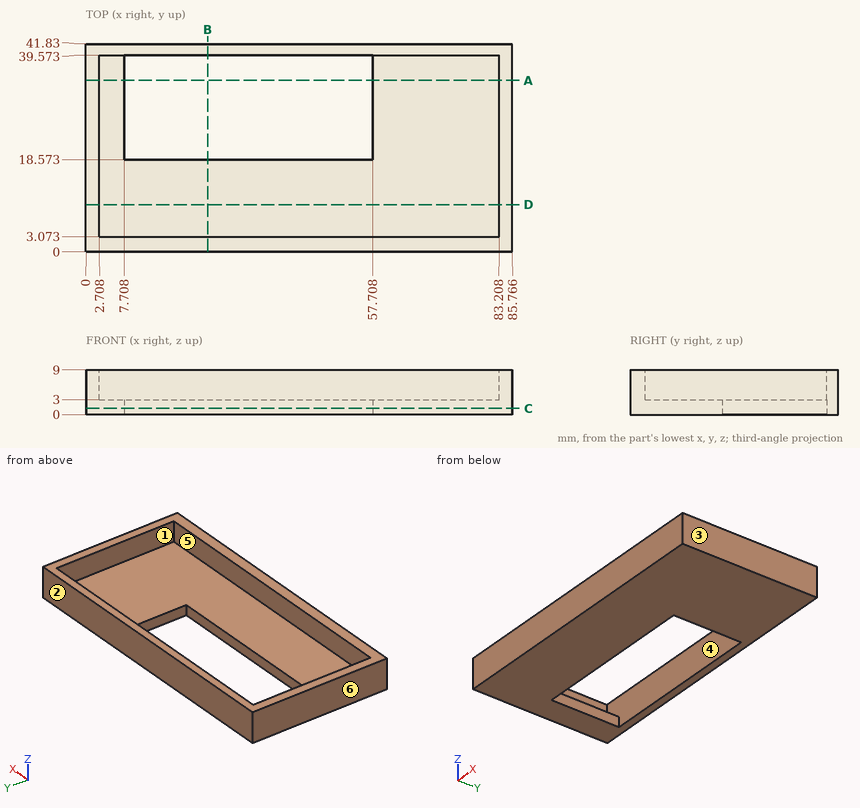
The figure shows three views and two pictorial views of one solid part (mm, origin at its lowest corner). Answer the questions. A direction names the side the tool comes from. Round coordinates to 2 decimals unless told otherwise and drop trailing zeros. Order: outer loops, then holes, each group sorted by start corner. A loop starts at its lowest first (then second) coordinate and runs counter-clockwise, first axis right, second up. Notation, with made-up numbers: (-40, -3.75) -> (6, -3.75) arc R16 cw to (6, 2.25) -> close; hole circle Ø9 at (7, 80.25). An arc over 180 degrees is marked (long way). Put each result on its own line as item: value.
Q1. Consider line 1 along X through (y, z) = (19, 7.5); line 2 along Y through (x, z) = (38.5, 7.5); line 3 along Y through (x, z) = (31.5, 1). Determine where each line is inside the solid, lowest interval first.
Results list:
line 1: 0 to 2.71, 83.21 to 85.77
line 2: 0 to 3.07, 39.57 to 41.83
line 3: 0 to 18.57, 39.57 to 41.83
Q2. Determine the mould class of the marked faces 3, 4, 5 and 6 for opening direction X: pulls with the +X half, pulls with the -X half, needs draft (parallel to the pull), parting line crosses it, or undercut.
Results list:
face 3: pulls with the +X half
face 4: undercut
face 5: undercut
face 6: pulls with the -X half
Q3. Section A-A, the plane y = 34.5 is taken. Write down the section's boundary in (x, z).
Results list:
outline: (0, 0) -> (7.71, 0) -> (7.71, 3) -> (2.71, 3) -> (2.71, 9) -> (0, 9) -> close; (57.71, 0) -> (85.77, 0) -> (85.77, 9) -> (83.21, 9) -> (83.21, 3) -> (57.71, 3) -> close
Q4. Section C-C, the plane z = 1.25 is taken. Write down the section's boundary in (x, y).
Results list:
outline: (0, 0) -> (85.77, 0) -> (85.77, 41.83) -> (0, 41.83) -> close; hole (7.71, 18.57) -> (57.71, 18.57) -> (57.71, 39.57) -> (7.71, 39.57) -> close
Q5. Section B-B, the plane x = 24.5 is taken. Write down the section's boundary in (y, z).
Results list:
outline: (0, 0) -> (18.57, 0) -> (18.57, 3) -> (3.07, 3) -> (3.07, 9) -> (0, 9) -> close; (39.57, 0) -> (41.83, 0) -> (41.83, 9) -> (39.57, 9) -> close
Q6. Which of the six approach directions +Z, -Z, +X, -X, +Y, -Y give full straight-line access (tool end or side, diameter ignored) to the marked faces 1 and 2?
Results list:
face 1: +Z
face 2: +Z, -Z, +X, -X, +Y
Q7. Section D-D, the plane y = 9.5 is taken. Write down the section's boundary in (x, z), and give its area (3 significant figures).
Results list:
outline: (0, 0) -> (85.77, 0) -> (85.77, 9) -> (83.21, 9) -> (83.21, 3) -> (2.71, 3) -> (2.71, 9) -> (0, 9) -> close
area: 289 mm^2
Q8. Each of these flat-tipped pins is pushed along its axis until it touches: P1, Ø1.8, axis at y = 19, z = 6.5, coming from the -X side; P2, Ø6, axis at x = 62.5, y = 30.5, coming from the +Z side. Where does it stop, or does it pass through?
Results list:
P1: x = 0
P2: z = 3
